```python
from build123d import *

# Parameters (mm, degrees)
SKETCH_1_R      = 1.6
EXTRUDE_1_DEPTH = 12


with BuildPart() as part:
    # 草图1 → 凸台-拉伸1 (new body)
    with BuildSketch(Plane.XY):
        with BuildLine():
            ThreePointArc((-1.5, 2.123676058), (-2.6, 0), (-1.5, -2.123676058))
            Line((-1.5, -2.123676058), (-1.5, -17))
            ThreePointArc((-1.5, -17), (0, -18.5), (1.5, -17))
            Line((1.5, -17), (1.5, -2.123676058))
            ThreePointArc((1.5, -2.123676058), (2.6, 0), (1.5, 2.123676058))
            Line((1.5, 2.123676058), (1.5, 5))
            ThreePointArc((1.5, 5), (0, 6.5), (-1.5, 5))
            Line((-1.5, 5), (-1.5, 2.123676058))
        make_face()
        Circle(SKETCH_1_R, mode=Mode.SUBTRACT)
    extrude(amount=EXTRUDE_1_DEPTH)


solid = part.part
```
The listing builds one solid part. Answer for the finished solid, in the listing's coordinates (mm). A direction names the side the tool comes from. Coordinates: 2 decimals unless noted, no trailing zeros. Write each loop counter-clockwise with the first axis right and the second up, starting at its lowest first coordinate (ties: lowest second). Pieces come first, ordered by that corner, then holes. Notation, with made-up numbers: (53, 80.5) -> (85, 80.5) arc R31 ccw to (85, 110.5) -> close; hole circle Ø8 at (-13.5, -37.75). An arc over 180 degrees is marked (long way). Write each question's results on one line, items separated by ' | '. Start each with the question number.
1) Flat-ended cylindrical pins translate along their axes: pin 1 Ø1.4 at (y, z) = (3.5, 5) entering from +X; pin 2 Ø3 at (y, z) = (4, 4.5) entering from -X; pin 3 Ø1 at (x, z) = (-1.5, 7.5) entering from -Y. Find the tip coordinate at first contact, or state that the pin passes through.
2) For a pull along X with two mould halves and no side action, classify faces 1 (the flat face through (0, -6, 12)), 2 (the cylindrical face through (-1.27, -0.97, 5.92)), 3 (the cylindrical face through (-2.6, 0, 5.9)) as +X half, -X half, draft (parallel to the pull), parting line (faces both ways), or undercut.
3) Straight lines are drawn through the part: probe 1 along Y at (x, z) = (0, 4.5); probe 2 along X at (y, z) = (-2.75, 10); probe 3 along Y at (x, z) = (1.3, 2). For each, find the intervals that lie inside material, in ascending order.
4) A cutting plane is placed at A-A (y = 0). Determine the outline of the cut face in (x, z), then the cut area to 3 significant figures.
5) A cutting plane is placed at C-C (z = 1.5). Determine the outline of the cut face in (x, y), then the cut area to 3 significant figures.
6) A tool of negligible diameter and unlimited length cuts with its end or side. For faces 4 (the flat face through (1.5, -10, 6)), 5 (the flat face through (1.5, 4, 6)), 6 (the flat face through (-1.5, -9, 6)), from which of +Z, -Z, +X, -X, +Y, -Y can it reach the whole face along a straight path? Write none if from no direction.
7) A cutting plane is placed at B-B (x = 0). Determine the outline of the cut face in (y, z).
8) A cutting plane is placed at D-D (y = 4.75). Determine the outline of the cut face in (x, z), then the cut area to 3 significant figures.
Values follow:
1) pin 1: x = 1.5 | pin 2: x = -1.5 | pin 3: y = -18.12
2) face 1: draft | face 2: undercut | face 3: -X half
3) probe 1: -18.5 to -1.6, 1.6 to 6.5 | probe 2: -1.5 to 1.5 | probe 3: -17.75 to -0.93, 0.93 to 5.75
4) outline: (-2.6, 0) -> (-1.6, 0) -> (-1.6, 12) -> (-2.6, 12) -> close; (1.6, 0) -> (2.6, 0) -> (2.6, 12) -> (1.6, 12) -> close | area: 24.0 mm²
5) outline: (-1.5, -17) arc R1.5 ccw to (1.5, -17) -> (1.5, -2.12) arc R2.6 ccw to (1.5, 2.12) -> (1.5, 5) arc R1.5 ccw to (-1.5, 5) -> (-1.5, 2.12) arc R2.6 ccw to (-1.5, -2.12) -> close; hole circle Ø3.2 at (0, 0) | area: 71.6 mm²
6) face 4: +Z, -Z, +X, -Y | face 5: +Z, -Z, +X, +Y | face 6: +Z, -Z, -X, -Y
7) outline: (-18.5, 0) -> (-1.6, 0) -> (-1.6, 12) -> (-18.5, 12) -> close; (1.6, 0) -> (6.5, 0) -> (6.5, 12) -> (1.6, 12) -> close
8) outline: (-1.5, 0) -> (1.5, 0) -> (1.5, 12) -> (-1.5, 12) -> close | area: 36.0 mm²
